from build123d import *

# Parameters (mm, degrees)
SKETCH1_W                       = 156
SKETCH1_H                       = 50
BOSS_EXTRUDE1_DEPTH             = 12.7
SKETCH2_W                       = 9.525
SKETCH2_H                       = 50
BOSS_EXTRUDE2_DEPTH             = 120
BOSS_EXTRUDE2_DIRECTION_2_REACH = 84.887
SKETCH3_R                       = 1.25
CUT_EXTRUDE1_DEPTH              = 214.250539272


with BuildPart() as part:
    # Sketch1 → Boss-Extrude1 (new body)
    with BuildSketch(Plane(origin=(0, 0, 0), x_dir=(1, 0, 0), z_dir=(0, 1, 0))):
        Rectangle(SKETCH1_W, SKETCH1_H)
    extrude(amount=BOSS_EXTRUDE1_DEPTH)

    # Sketch2 → Boss-Extrude2 (add)
    with BuildSketch(Plane(origin=(0, 12.7, 0), x_dir=(1, 0, 0), z_dir=(0, 1, 0))):
        with Locations((-77.7625, 0)):
            Rectangle(SKETCH2_W, SKETCH2_H)
        with Locations((77.7625, 0)):
            Rectangle(SKETCH2_W, SKETCH2_H)
    extrude(amount=BOSS_EXTRUDE2_DEPTH)

    # Boss-Extrude2 direction 2: up to this face of the body (flat: up to its plane)
    boss_extrude2_direction_2_end = Plane(part.part.faces().sort_by_distance((0, 0, 0))[0])
    # Sketch2 → Boss-Extrude2 direction 2 (add, up to the picked face)
    with BuildSketch(Plane(origin=(0, 12.7, 0), x_dir=(1, 0, 0), z_dir=(0, 1, 0)), mode=Mode.PRIVATE) as boss_extrude2_direction_2_sk1:
        with Locations((-77.7625, 0)):
            Rectangle(SKETCH2_W, SKETCH2_H)
    boss_extrude2_direction_2_tool1 = split(extrude(boss_extrude2_direction_2_sk1.sketch, amount=-BOSS_EXTRUDE2_DIRECTION_2_REACH, mode=Mode.PRIVATE), bisect_by=boss_extrude2_direction_2_end, keep=Keep.BOTH, mode=Mode.PRIVATE)
    # Sketch2 → Boss-Extrude2 direction 2 (add, up to the picked face)
    with BuildSketch(Plane(origin=(0, 12.7, 0), x_dir=(1, 0, 0), z_dir=(0, 1, 0)), mode=Mode.PRIVATE) as boss_extrude2_direction_2_sk2:
        with Locations((77.7625, 0)):
            Rectangle(SKETCH2_W, SKETCH2_H)
    boss_extrude2_direction_2_tool2 = split(extrude(boss_extrude2_direction_2_sk2.sketch, amount=-BOSS_EXTRUDE2_DIRECTION_2_REACH, mode=Mode.PRIVATE), bisect_by=boss_extrude2_direction_2_end, keep=Keep.BOTH, mode=Mode.PRIVATE)
    add(boss_extrude2_direction_2_tool1.solids().sort_by(Axis((-77.7625, 12.7, 0), (0, -1, 0)))[0])
    add(boss_extrude2_direction_2_tool2.solids().sort_by(Axis((77.7625, 12.7, 0), (0, -1, 0)))[0])

    # Sketch3 → Cut-Extrude1 (cut, through all)
    with BuildSketch(Plane(origin=(82.525, 0, 0), x_dir=(0, 0, -1), z_dir=(1, 0, 0))):
        with Locations((0, 122.7)):
            Circle(SKETCH3_R)
        with Locations((0, 97.7)):
            Circle(SKETCH3_R)
        with Locations((0, 72.7)):
            Circle(SKETCH3_R)
        with Locations((0, 47.7)):
            Circle(SKETCH3_R)
        with Locations((0, 22.7)):
            Circle(SKETCH3_R)
    extrude(amount=-CUT_EXTRUDE1_DEPTH, mode=Mode.SUBTRACT)


solid = part.part
Geometry: final body of the model. Coordinates: model frame, mm. A direction names the side the tool comes from. Coordinates: 2 decimals unless noted, no trailing zeros. Order: outer loops, then holes, each group sorted by start corner. A loop starts at its lowest first (then second) coordinate and runs counter-clockwise, first axis right, second up. Notation, with made-up numbers: M -7,44 L 17,44 A15 ccw 17,73 Z; hole C 68.25,43.25 d4. An arc over 180 degrees is marked long. One line per question, with ' | ' between items. Start each with the question number.
Item 1: Cut plane A-A, the plane y = 33. Return the cut outline in (x, z) (3 decimals), then the cut area to 4 significant figures.
Item 2: Cut plane B-B, the plane z = 7. Return the cut outline in (x, y) (3 decimals).
Item 3: Cut plane C-C, the plane x = -50. Return the cut outline in (y, z), then the cut area to 3 significant figures.
Item 4: Set-up query: faces 4 (the flat face through (-73, 72, 6)), 5 (the flat face through (-6, 8, -25)). Return all of +Z, -Z, +X, -X, +Y, -Y with unobstructed straight access to the full face (end or side cutting, diameter ignored); none if empty.
Item 5: Ray query, probe 1 along Y at (x, z) = (76.25, 0); probe 2 along X at (y, z) = (26.5, -10) (3 decimals); probe 3 along Z at (x, y) = (79.25, 122.7). Return the intervals inside material, ascending. Write a range as [from, to].
Item 6: Pin query (flat end, axial travel): pin 1 Ø2 at (y, z) = (72.7, 0) entering from +X; pin 2 Ø3 at (x, z) = (-6.5, 13) entering from +Y. Return the tip coordinate at first contact, or that it passes through.
Item 7: Draft query along X for faces 1 (the flat face through (-1, 12.7, 0)), 2 (the flat face through (-78, 132.7, 0)), 3 (the flat face through (82.525, 65, 0)). Return one class per face: released by +X, released by -X, zero draft, split by the parting line, or undercut.
A:
1) outline: M -82.525,-25 L -73,-25 L -73,25 L -82.525,25 Z; M 73,-25 L 82.525,-25 L 82.525,25 L 73,25 Z | area: 952.5 mm2
2) outline: M -82.525,0 L 82.525,0 L 82.525,132.7 L 73,132.7 L 73,12.7 L -73,12.7 L -73,132.7 L -82.525,132.7 Z
3) outline: M 0,-25 L 12.7,-25 L 12.7,25 L 0,25 Z | area: 635 mm2
4) face 4: +Z, -Z, +Y | face 5: -Z, +X, -X, +Y, -Y
5) probe 1: y = [0, 21.45], [23.95, 46.45], [48.95, 71.45], [73.95, 96.45], [98.95, 121.45], [123.95, 132.7] | probe 2: x = [-82.525, -73], [73, 82.525] | probe 3: z = [-25, -1.25], [1.25, 25]
6) pin 1: passes through | pin 2: stops at y = 12.7
7) face 1: undercut | face 2: zero draft | face 3: released by +X
